For this review, take the finished solid that the model builds, in its own axes (mm). Face numbers are marked on the shaded views. A direction names the side the tool comes from. Give positions to 0.01 mm unless a question says otherwise; leave off trailing zeros. Loops run counter-clockwise (first coordinate to the right, second up) from the corner with the lowest first, then second, coordinate; pieces in that order, holes last.
```python
from build123d import *

# Parameters (mm, degrees)
SKETCH1_W              = 250
SKETCH1_H              = 25
BOSS_EXTRUDE1_DEPTH    = 10
CUT_EXTRUDE1_REACH     = 253.446
SKETCH2_R              = 2.15
FILLET1_R              = 12.5
SKETCH3_R              = 2.25
CUT_EXTRUDE2_DEPTH     = 252.445819214
CUT_EXTRUDE5_REACH     = 253.446
SKETCH5_W              = 7.3
SKETCH5_H              = 4
SKETCH6_R              = 10
CUT_EXTRUDE6_DEPTH     = 5
CUT_EXTRUDE7_REACH     = 253.297
SKETCH7_R              = 1.65
CUT_EXTRUDE8_START     = -3.2
CUT_EXTRUDE8_OUTLINE_W = 6
CUT_EXTRUDE8_OUTLINE_H = 6
CUT_EXTRUDE8_DEPTH     = 6.4
SKETCH9_R              = 3
CUT_EXTRUDE9_DEPTH     = 2
CUT_EXTRUDE10_DEPTH    = 252.445819214
SKETCH11_R             = 2.25
CUT_EXTRUDE11_DEPTH    = 158.321327226


# Read off the part's stored shape, not the designer's step: Cut-Extrude8
with BuildPart() as part:
    # Sketch1 → Boss-Extrude1 (new body)
    with BuildSketch(Plane(origin=(0, 0, 0), x_dir=(1, 0, 0), z_dir=(0, 1, 0))):
        with Locations((125, 12.5)):
            Rectangle(SKETCH1_W, SKETCH1_H)
    extrude(amount=BOSS_EXTRUDE1_DEPTH)

    # Sketch2 → Cut-Extrude1 (cut, up to next)
    with BuildSketch(Plane(origin=(0, 10, 0), x_dir=(1, 0, 0), z_dir=(0, 1, 0)), mode=Mode.PRIVATE) as cut_extrude1_sk1:
        with Locations(Location((12.5, 12.5, 0), (0, 0, 270))):
            Circle(SKETCH2_R)
    cut_extrude1_tool1 = extrude(cut_extrude1_sk1.sketch, amount=-CUT_EXTRUDE1_REACH, mode=Mode.PRIVATE) & part.part
    add(cut_extrude1_tool1.solids().sort_by_distance((12.5, 10, -12.5))[0], mode=Mode.SUBTRACT)

    # Fillet1
    fillet1_edges = [part.edges().sort_by_distance(p)[0] for p in [
        (0, 5, 0),
        (0, 5, -25),
    ]]
    fillet(fillet1_edges, radius=FILLET1_R - 0.0001)  # a hair under: the kernel refuses the full size

    # Sketch3 → Cut-Extrude2 (cut, through all)
    with BuildSketch(Plane(origin=(0, 0, -25), x_dir=(-1, 0, 0), z_dir=(0, 0, -1))):
        with Locations((-244.5, 5)):
            Circle(SKETCH3_R)
        with Locations((-230.5, 5)):
            Circle(SKETCH3_R)
    extrude(amount=-CUT_EXTRUDE2_DEPTH, mode=Mode.SUBTRACT)

    # Sketch5 → Cut-Extrude5 (cut, up to next)
    with BuildSketch(Plane(origin=(0, 10, 0), x_dir=(1, 0, 0), z_dir=(0, 1, 0)), mode=Mode.PRIVATE) as cut_extrude5_sk1:
        with Locations((244.5, 19)):
            Rectangle(SKETCH5_W, SKETCH5_H)
    cut_extrude5_tool1 = extrude(cut_extrude5_sk1.sketch, amount=-CUT_EXTRUDE5_REACH, mode=Mode.PRIVATE) & part.part
    # Sketch5 → Cut-Extrude5 (cut, up to next)
    with BuildSketch(Plane(origin=(0, 10, 0), x_dir=(1, 0, 0), z_dir=(0, 1, 0)), mode=Mode.PRIVATE) as cut_extrude5_sk2:
        with Locations((244.5, 6)):
            Rectangle(SKETCH5_W, SKETCH5_H)
    cut_extrude5_tool2 = extrude(cut_extrude5_sk2.sketch, amount=-CUT_EXTRUDE5_REACH, mode=Mode.PRIVATE) & part.part
    # Sketch5 → Cut-Extrude5 (cut, up to next)
    with BuildSketch(Plane(origin=(0, 10, 0), x_dir=(1, 0, 0), z_dir=(0, 1, 0)), mode=Mode.PRIVATE) as cut_extrude5_sk3:
        with Locations((230.5, 19)):
            Rectangle(SKETCH5_W, SKETCH5_H)
    cut_extrude5_tool3 = extrude(cut_extrude5_sk3.sketch, amount=-CUT_EXTRUDE5_REACH, mode=Mode.PRIVATE) & part.part
    # Sketch5 → Cut-Extrude5 (cut, up to next)
    with BuildSketch(Plane(origin=(0, 10, 0), x_dir=(1, 0, 0), z_dir=(0, 1, 0)), mode=Mode.PRIVATE) as cut_extrude5_sk4:
        with Locations((230.5, 6)):
            Rectangle(SKETCH5_W, SKETCH5_H)
    cut_extrude5_tool4 = extrude(cut_extrude5_sk4.sketch, amount=-CUT_EXTRUDE5_REACH, mode=Mode.PRIVATE) & part.part
    add(cut_extrude5_tool1.solids().sort_by_distance((244.5, 10, -19))[0], mode=Mode.SUBTRACT)
    add(cut_extrude5_tool2.solids().sort_by_distance((244.5, 10, -6))[0], mode=Mode.SUBTRACT)
    add(cut_extrude5_tool3.solids().sort_by_distance((230.5, 10, -19))[0], mode=Mode.SUBTRACT)
    add(cut_extrude5_tool4.solids().sort_by_distance((230.5, 10, -6))[0], mode=Mode.SUBTRACT)

    # Sketch6 → Cut-Extrude6 (cut)
    with BuildSketch(Plane.XZ):
        with Locations(Location((12.5, -12.5, 0), (0, 0, 270))):
            Circle(SKETCH6_R)
    extrude(amount=-CUT_EXTRUDE6_DEPTH, mode=Mode.SUBTRACT)

    # Sketch7 → Cut-Extrude7 (cut, up to next)
    with BuildSketch(Plane.XZ.offset(-5), mode=Mode.PRIVATE) as cut_extrude7_sk1:
        with Locations(Location((12.5, -6, 0), (0, 0, 270))):
            Circle(SKETCH7_R)
    cut_extrude7_tool1 = extrude(cut_extrude7_sk1.sketch, amount=-CUT_EXTRUDE7_REACH, mode=Mode.PRIVATE) & part.part
    # Sketch7 → Cut-Extrude7 (cut, up to next)
    with BuildSketch(Plane.XZ.offset(-5), mode=Mode.PRIVATE) as cut_extrude7_sk2:
        with Locations(Location((19, -12.5, 0), (0, 0, 270))):
            Circle(SKETCH7_R)
    cut_extrude7_tool2 = extrude(cut_extrude7_sk2.sketch, amount=-CUT_EXTRUDE7_REACH, mode=Mode.PRIVATE) & part.part
    # Sketch7 → Cut-Extrude7 (cut, up to next)
    with BuildSketch(Plane.XZ.offset(-5), mode=Mode.PRIVATE) as cut_extrude7_sk3:
        with Locations(Location((12.5, -19, 0), (0, 0, 270))):
            Circle(SKETCH7_R)
    cut_extrude7_tool3 = extrude(cut_extrude7_sk3.sketch, amount=-CUT_EXTRUDE7_REACH, mode=Mode.PRIVATE) & part.part
    # Sketch7 → Cut-Extrude7 (cut, up to next)
    with BuildSketch(Plane.XZ.offset(-5), mode=Mode.PRIVATE) as cut_extrude7_sk4:
        with Locations(Location((6, -12.5, 0), (0, 0, 270))):
            Circle(SKETCH7_R)
    cut_extrude7_tool4 = extrude(cut_extrude7_sk4.sketch, amount=-CUT_EXTRUDE7_REACH, mode=Mode.PRIVATE) & part.part
    add(cut_extrude7_tool1.solids().sort_by_distance((12.5, 5, -6))[0], mode=Mode.SUBTRACT)
    add(cut_extrude7_tool2.solids().sort_by_distance((19, 5, -12.5))[0], mode=Mode.SUBTRACT)
    add(cut_extrude7_tool3.solids().sort_by_distance((12.5, 5, -19))[0], mode=Mode.SUBTRACT)
    add(cut_extrude7_tool4.solids().sort_by_distance((6, 5, -12.5))[0], mode=Mode.SUBTRACT)

    # Cut-Extrude8 outline → Cut-Extrude8 (cut)
    with BuildSketch(Plane(origin=(0, 0, 0), x_dir=(0.707106781186548, 0, -0.707106781186547), z_dir=(0.707106781186547, 0, 0.707106781186548)).offset(CUT_EXTRUDE8_START)):
        with Locations((7, 2)):
            Rectangle(CUT_EXTRUDE8_OUTLINE_W, CUT_EXTRUDE8_OUTLINE_H)
    extrude(amount=CUT_EXTRUDE8_DEPTH, mode=Mode.SUBTRACT)

    # Sketch9 → Cut-Extrude9 (cut)
    with BuildSketch(Plane(origin=(0, 10, 0), x_dir=(1, 0, 0), z_dir=(0, 1, 0))):
        with Locations(Location((12.5, 19, 0), (0, 0, 270))):
            Circle(SKETCH9_R)
        with Locations(Location((19, 12.5, 0), (0, 0, 270))):
            Circle(SKETCH9_R)
        with Locations(Location((12.5, 6, 0), (0, 0, 270))):
            Circle(SKETCH9_R)
        with Locations(Location((6, 12.5, 0), (0, 0, 270))):
            Circle(SKETCH9_R)
    extrude(amount=-CUT_EXTRUDE9_DEPTH, mode=Mode.SUBTRACT)

    # Sketch10 → Cut-Extrude10 (cut, through all)
    with BuildSketch(Plane(origin=(0, 10, 0), x_dir=(1, 0, 0), z_dir=(0, 1, 0))):
        Polygon((95, 5), (155, 5), (155, 0), (250, 0), (250, 25), (155, 25), (155, 20), (95, 20), align=None)
    extrude(amount=-CUT_EXTRUDE10_DEPTH, mode=Mode.SUBTRACT)

    # Sketch11 → Cut-Extrude11 (cut, through all)
    with BuildSketch(Plane.XY):
        with Locations((150, 5)):
            Circle(SKETCH11_R)
        with Locations((140, 5)):
            Circle(SKETCH11_R)
        with Locations((130, 5)):
            Circle(SKETCH11_R)
        with Locations((120, 5)):
            Circle(SKETCH11_R)
        with Locations((110, 5)):
            Circle(SKETCH11_R)
    extrude(amount=-CUT_EXTRUDE11_DEPTH, mode=Mode.SUBTRACT)


solid = part.part
```
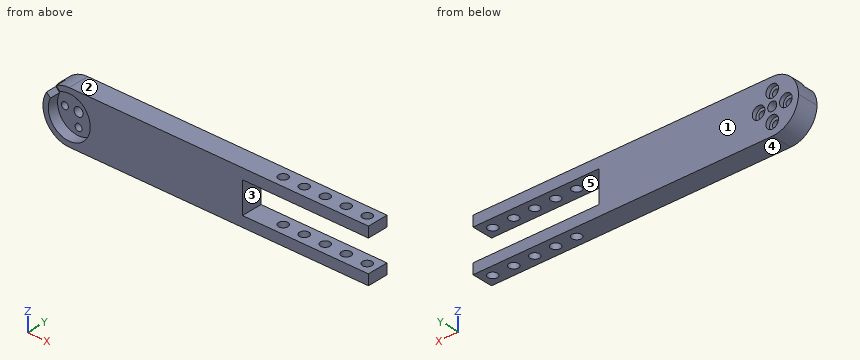
Item 1: Clearance check with flat-ended pins moving along their axes: pin 1 Ø3.5 at (x, y) = (120, 5) entering from +Z; pin 2 Ø6 at (x, z) = (12.5, -11) entering from -Y; pin 3 Ø3 at (y, z) = (3, -14) entering from +X; pin 4 Ø4.5 at (x, z) = (12.5, -6) entering from +Y. State where each tip first meets the part, or that it passes through.
Answer:
pin 1: passes through
pin 2: stops at y = 5
pin 3: stops at x = 95
pin 4: stops at y = 8
Item 2: The part is to be moulded in two halves that separate along Z. For the marked faces 1, 2 and 3, say which applies: released by +Z, released by -Z, zero draft, split by the parting line, or undercut.
Answer:
face 1: zero draft
face 2: released by +Z
face 3: undercut
Item 3: Take a section at B-B on x = 98. Give the boundary of the cut face in (y, z), and give its area (3 significant figures).
Answer:
outline: (0, -25) - (10, -25) - (10, -20) - (0, -20) - close; (0, -5) - (10, -5) - (10, 0) - (0, 0) - close
area: 100 mm2
Item 4: Take a section at C-C on x = 19. Give the boundary of the cut face in (y, z).
Answer:
outline: (0, -25) - (10, -25) - (10, -15.5) - (8, -15.5) - (8, -14.15) - (5, -14.15) - (5, -20.1) - (0, -20.1) - close; (0, -4.9) - (5, -4.9) - (5, -10.85) - (8, -10.85) - (8, -9.5) - (10, -9.5) - (10, 0) - (0, 0) - close
Item 5: Take a section at A-A on x = 130. Give the boundary of the cut face in (y, z).
Answer:
outline: (0, -25) - (2.75, -25) - (2.75, -20) - (0, -20) - close; (0, -5) - (2.75, -5) - (2.75, 0) - (0, 0) - close; (7.25, -25) - (10, -25) - (10, -20) - (7.25, -20) - close; (7.25, -5) - (10, -5) - (10, 0) - (7.25, 0) - close
Item 6: Tool access review of the marked faces 4 and 5: name each direction out of +Z, -Z, +X, -X, +Y, -Y from which nothing blocks a thin tool from reaching the whole face with its end or side.
Answer:
face 4: -Z, +X, -X, +Y, -Y
face 5: +X, +Y, -Y
Item 7: For L1, parallel to X at y = 9.3, z = -12.5; L2, parallel to Z at x = 143, y = 5.25; L3, parallel to X at y = 5.5, z = -11.25, list the stretches that pass through material, from the lowest coordinate up.
Answer:
L1: x = 0 to 3, 9 to 10.35, 14.65 to 16, 22 to 95
L2: z = -25 to -20, -5 to 0
L3: x = 0.06 to 4.92, 7.08 to 10.75, 14.25 to 17.92, 20.08 to 95
